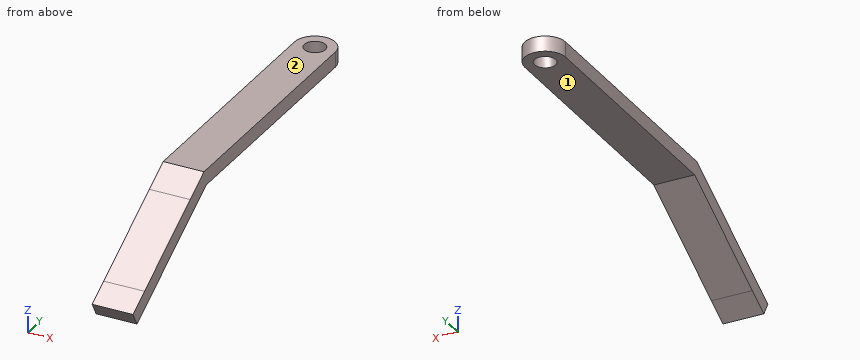
Autodesk Inventor part; units mm, degrees
ref_plane "YZ Plane" through (0, 0, 0) normal (1, 0, 0) x (0, 1, 0)
ref_plane "XZ Plane" through (0, 0, 0) normal (0, 1, 0) x (-1, 0, 0)
ref_plane "XY Plane" through (0, 0, 0) normal (0, 0, 1) x (1, 0, 0)
sketch "Sketch1" plane through (0, 0, 0) normal (0, 0, 1) x (1, 0, 0)
  circle A0 centre (0, 0) radius 2.0828
  dimension "d0" = 4.1656
sketch "Sketch2" plane through (0, 0, 0) normal (0, 0, 1) x (1, 0, 0)
  circle A0 centre (0, 0) radius 4
  dimension "d1" = 8
extrude "Extrusion1" add sketch "Sketch2" along normal blind 3
sketch "Sketch3" plane through (0, 0, 3) normal (0, 0, 1) x (1, 0, 0)
  circle A0 centre (0, 0) radius 4
  line L0 (-4, 0) -> (4, 0)
  line L1 (4, 0) -> (4, -70)
  line L2 (4, -70) -> (-4, -70)
  line L3 (-4, -70) -> (-4, 0)
  dimension "d4" = 70
extrude "Extrusion2" add sketch "Sketch3" against normal blind 3 contours L1 L2 L3 A0
extrude "Extrusion3" cut sketch "Sketch1" along normal blind 5
sketch "Sketch4" plane through (-4, -70, 3) normal (-1, 0, 0) x (0, 0, 1)
  line L0 (-3, 0) -> (-3, 70)
  line L1 (-3, 0) -> (-15.5, 0)
  line L2 (-15.5, 0) -> (-3, 21.5912)
  line L3 (-15.5, 0) -> (-12.9037, -1.5031)
  line L4 (-12.9037, -1.5031) -> (-3, 15.6035)
  dimension "d9" = 12.5
  dimension "d10" = 3
extrude "Extrusion4" add sketch "Sketch4" against normal blind 8 contours L4 L1 L2 L0 | L4 L3 L1
sketch "Sketch5" plane through (-4, -70, 3) normal (-1, 0, 0) x (0, 0, 1)
  line L0 (-3, 15.6035) -> (-12.9037, -1.5031)
  line L1 (-3.8073, 14.2091) -> (2.2743, 24.7138)
  line L2 (2.2743, 24.7138) -> (2.8326, -0.03)
  line L3 (2.8326, -0.03) -> (-4.8388, -0.2031)
  line L4 (-4.8388, -0.2031) -> (-3.8073, 14.2091)
  point P0 (-3, 70)
extrude "Extrusion5" cut sketch "Sketch5" against normal blind 8
sketch "Sketch6" plane through (-4, -70, -12.5) normal (0, -0.8654, -0.501) x (1, 0, 0)
  line L0 (0, 0) -> (0, 3)
  line L1 (8, 0) -> (0, 0)
  line L2 (0, 0) -> (8, 0)
  line L3 (8, 0) -> (8, 3)
  line L4 (8, 3) -> (0, 3)
  line L5 (0, 3) -> (0, 0)
  point P0 (4, -24.2544)
extrude "Extrusion6" add sketch "Sketch6" along normal blind 5
properties part number "Thumb"
Source: CAD feature listing. Evaluate the final solid. Frame: model axes, mm. Face numbers are marked on the shaded views. A direction names the side the tool comes from. Coordinates: 2 decimals unless noted, no trailing zeros. Order: outer loops, then holes, each group sorted by start corner. A loop starts at its lowest first (then second) coordinate and runs counter-clockwise, first axis right, second up. Notation, with made-up numbers: (70.25, 81) - (94.25, 81) arc R30 ccw to (94.25, 113) - close; hole circle Ø4 at (-32.5, 23.5). An arc over 180 degrees is marked (long way). One line per item, written item: value.
1) Cut plane C-C on y = -21.5. Output: boundary loops of the cut face in (x, z).
Computed values:
outline: (-4, 0) - (4, 0) - (4, 3) - (-4, 3) - close
2) Contact query for flat-ended pins moving along their axis: pin 1 (3 mm diameter, centred on x = -0.5, z = -10.5, fed in from -Y); pin 2 (4 mm diameter, centred on x = -2, y = -20, fed in from -Z); pin 3 (1 mm diameter, centred on x = 1.5, z = -2.5, fed in from -Y). Output: stop coordinate, or through.
Computed values:
pin 1: stops at y = -75.12
pin 2: stops at z = 0
pin 3: stops at y = -59.58
3) Reachability of the marked faces 1 and 2 from +Z, -Z, +X, -X, +Y, -Y: full face, straight path, thin tool, end or side. Return the list, or none.
Computed values:
face 1: -Z, +X, -X, +Y
face 2: +Z, +X, -X, +Y, -Y
4) Cut plane D-D on z = -2.5. Output: boundary loops of the cut face in (x, y), plus the area to 3 significant figures.
Computed values:
outline: (-4, -58.71) - (4, -58.71) - (4, -52.73) - (-4, -52.73) - close
area: 47.9 mm^2
5) Cut plane B-B on z = 2.25. Output: boundary loops of the cut face in (x, y), plus the area to 3 significant figures.
Computed values:
outline: (-4, -50.51) - (4, -50.51) - (4, 0) arc R4 ccw to (-4, 0) - close; hole circle Ø4.17 at (0, 0)
area: 416 mm^2
6) Ray query, line 1 (X direction, y = 0, z = 0.85); line 2 (X direction, y = 1.5, z = 1.5); line 3 (Y direction, x = 0, z = 0.7). Return the intervals inside material, ascending. Write a range as [from, to].
Computed values:
line 1: x = [-4, -2.08], [2.08, 4]
line 2: x = [-3.71, -1.45], [1.45, 3.71]
line 3: y = [-53.19, -2.08], [2.08, 4]
